```python
from build123d import *

# Parameters (mm, degrees)
F1_DEPTH = 2.5
F0_W     = 5
F0_H     = 5
F2_DEPTH = 20
F3_W     = 50
F3_H     = 130
F4_DEPTH = 2.5


with BuildPart() as f1:
    # F0 (on Top) → F1 (new body)
    with BuildSketch(Plane.XY):
        Polygon((17, 60), (17, 65), (-17, 65), (-17, 60), (-22, 60), (-22, -58), (22, -58), (22, 60), align=None)
    extrude(amount=F1_DEPTH)

    # F0 (on Top) → F2 (join)
    with BuildSketch(Plane.XY):
        with Locations((19.5, 62.5)):
            Rectangle(F0_W, F0_H)
        Polygon((25, -65), (25, 65), (22, 65), (22, 60), (22, -58), (-22, -58), (-22, 60), (-22, 65), (-25, 65), (-25, -65), align=None)
        with Locations((-19.5, 62.5)):
            Rectangle(F0_W, F0_H)
    extrude(amount=F2_DEPTH)

    # F3 (on face) → F4 (join)
    with BuildSketch(Plane.XY.offset(20)):
        Rectangle(F3_W, F3_H)
    extrude(amount=F4_DEPTH)


solid = f1.part
```
Can you work these out from the model? Positions are in its coordinate system, mm. A direction names the side the tool comes from. Coordinates: 2 decimals unless noted, no trailing zeros. Loops run counter-clockwise (first coordinate to the right, second up) from the corner with the lowest first, then second, coordinate; pieces in that order, holes last. Notation, with made-up numbers: (58.25, 5.5) -> (102.25, 5.5) arc R23 ccw to (102.25, 38.5) -> close; hole circle Ø3 at (37.25, 42.25). An arc over 180 degrees is marked (long way). Put each result on its own line as item: value. Start each with the question number.
Q1. I want a section at B-B (x = 19). Write out the boundary of the cut face in (y, z).
Q2. I'm going to push flat-ended pins straight in: P1, Ø3, axis at x = -16, z = 10.5, coming from the +Y side; P2, Ø1, axis at x = 4, z = 8.5, coming from the +Y side. Where does each tip first touch, or does it pass through?
Q3. If I drill on line 1 (X direction, y = 32, z = 15.75); line 2 (Z direction, x = 18.5, y = -3); line 3 (Y direction, x = 20, z = 10), over which ranges is the centre line in solid material (lowest first)? Write a range as [from, to].
Q4. I want a section at D-D (x = -12). Write out the boundary of the cut face in (y, z).
Q5. Thinking about a two-plate mould opening in Y: for faces 1 (the face through (-17, 62, 11)), 2 (the face through (0, 4, 2.5)), 3 (the face through (-6, 65, 1)), which applies, pulls with the +Y half, pulls with the -Y half, needs draft (parallel to the pull), parting line crosses it, or undercut?
Q6. I want a section at C-C (z = 14). Write out the boundary of the cut face in (x, y).
Q7. For faces 4 (the face through (-25, -1, 11)), 5 (the face through (17, 62, 11)), 6 (the face through (0, -58, 11)), which set-ups out of +Z, -Z, +X, -X, +Y, -Y let a thin tool reach every point of the face, with its end or its side?
Q8. I want a section at A-A (y = 42). Write out the boundary of the cut face in (x, z), plus the area to 3 significant figures.
Taken from the geometry:
1. outline: (-65, 0) -> (65, 0) -> (65, 22.5) -> (-65, 22.5) -> close; hole (-58, 2.5) -> (60, 2.5) -> (60, 20) -> (-58, 20) -> close
2. P1: stops at y = 65
2. P2: stops at y = -58
3. line 1: x = [-25, -22], [22, 25]
3. line 2: z = [0, 2.5], [20, 22.5]
3. line 3: y = [-65, -58], [60, 65]
4. outline: (-65, 0) -> (65, 0) -> (65, 2.5) -> (-58, 2.5) -> (-58, 20) -> (65, 20) -> (65, 22.5) -> (-65, 22.5) -> close
5. face 1: needs draft
5. face 2: undercut
5. face 3: pulls with the +Y half
6. outline: (-25, -65) -> (25, -65) -> (25, 65) -> (17, 65) -> (17, 60) -> (22, 60) -> (22, -58) -> (-22, -58) -> (-22, 60) -> (-17, 60) -> (-17, 65) -> (-25, 65) -> close
7. face 4: +Z, -Z, -X, +Y, -Y
7. face 5: +Y
7. face 6: none
8. outline: (-25, 0) -> (25, 0) -> (25, 22.5) -> (-25, 22.5) -> close; hole (-22, 2.5) -> (22, 2.5) -> (22, 20) -> (-22, 20) -> close
8. area: 355 mm2
